The listing builds one solid part. Answer for the finished solid, in the listing's coordinates (mm). A direction names the side the tool comes from. Round coordinates to 2 decimals unless told otherwise and drop trailing zeros. Order: outer loops, then holes, each group sorted by start corner. A loop starts at its lowest first (then second) coordinate and runs counter-clockwise, first axis right, second up. Notation, with made-up numbers: (51, 87) -> (104, 87) arc R17 ccw to (104, 99) -> close; hole circle Ø10 at (-34.75, 65). An arc over 180 degrees is marked (long way). Answer in a Markdown table with one row per item. Add a question column.
Autodesk Inventor part; units mm, degrees
ref_plane "YZ Plane" through (0, 0, 0) normal (1, 0, 0) x (0, 1, 0)
ref_plane "XZ Plane" through (0, 0, 0) normal (0, 1, 0) x (-1, 0, 0)
ref_plane "XY Plane" through (0, 0, 0) normal (0, 0, 1) x (1, 0, 0)
sketch "Sketch1" plane through (0, 0, 0) normal (0, 0, 1) x (1, 0, 0)
  line L0 (-11.5482, -7.036) -> (-11.5482, 82.964)
  line L1 (-11.5482, 82.964) -> (68.4518, 82.964)
  line L2 (68.4518, 82.964) -> (68.4518, -7.036)
  line L3 (68.4518, -7.036) -> (-11.5482, -7.036)
  line L4 (5.9518, 27.964) -> (5.9518, 67.964)
  line L5 (5.9518, 67.964) -> (50.9518, 67.964)
  line L6 (50.9518, 67.964) -> (50.9518, 27.964)
  line L7 (50.9518, 27.964) -> (43.4518, 27.964)
  line L8 (43.4518, 27.964) -> (43.4518, -2.036)
  line L9 (43.4518, -2.036) -> (13.4518, -2.036)
  line L10 (13.4518, -2.036) -> (13.4518, 27.964)
  line L11 (13.4518, 27.964) -> (5.9518, 27.964)
  point P0 (0, 0)
  dimension "d0" = 90
  dimension "d1" = 80
  dimension "d2" = 90
  dimension "d3" = 45
  dimension "d4" = 40
  dimension "d5" = 7.5
  dimension "d6" = 30
  dimension "d7" = 17.5
  dimension "d8" = 15
  dimension "d9" = 30
extrude "Extrusion1" add sketch "Sketch1" against normal blind 35
properties part number "BT002_Matrize"
Item 1: The part is cut by section A-A, the plane x = 16. Give the vertices of the cut face in (y, z), and give its area (3 significant figures).
Item 2: The part is cut by section C-C, the plane z = -20.5. Give the vertices of the cut face in (x, y).
Item 3: A tool of negligible diameter and unlimited length cuts with its end or side. For faces 1 (the face through (13.452, 13, -17)), 2 (the face through (29, -7.036, -17)), from which of +Z, -Z, +X, -X, +Y, -Y can it reach the whole face along a straight path? Write none if from no direction.
Item 4: For a pull along X with two mould halves and no side action, classify faces 3 (the face through (68.452, 39, -17)), 4 (the face through (-11.548, 37, -17)), 5 (the face through (47, 27.964, -17)) as released by +X, released by -X, zero draft, split by the parting line, or undercut.
Item 5: The part is cut by section B-B, the plane y = 41. Give the vertices of the cut face in (x, z), and give its area (4 significant figures).
Item 6: Find the intervals of material crossed by probe 1 along Y at (x, z) = (44, -6); probe 2 along Y at (x, z) = (28, -26.5); probe 3 along X at (y, z) = (8.5, -18.5), in increasing order. Write a range as [from, to].
Resolved:
| question | item | result |
|---|---|---|
| 1 | outline | (-7.04, -35) -> (-2.04, -35) -> (-2.04, 0) -> (-7.04, 0) -> close; (67.96, -35) -> (82.96, -35) -> (82.96, 0) -> (67.96, 0) -> close |
| 1 | area | 700 mm2 |
| 2 | outline | (-11.55, -7.04) -> (68.45, -7.04) -> (68.45, 82.96) -> (-11.55, 82.96) -> close; hole (5.95, 27.96) -> (13.45, 27.96) -> (13.45, -2.04) -> (43.45, -2.04) -> (43.45, 27.96) -> (50.95, 27.96) -> (50.95, 67.96) -> (5.95, 67.96) -> close |
| 3 | face 1 | +Z, -Z |
| 3 | face 2 | +Z, -Z, +X, -X, -Y |
| 4 | face 3 | released by +X |
| 4 | face 4 | released by -X |
| 4 | face 5 | undercut |
| 5 | outline | (-11.55, -35) -> (5.95, -35) -> (5.95, 0) -> (-11.55, 0) -> close; (50.95, -35) -> (68.45, -35) -> (68.45, 0) -> (50.95, 0) -> close |
| 5 | area | 1,225 mm2 |
| 6 | probe 1 | [-7.04, 27.96], [67.96, 82.96] |
| 6 | probe 2 | [-7.04, -2.04], [67.96, 82.96] |
| 6 | probe 3 | [-11.55, 13.45], [43.45, 68.45] |
